Autodesk Inventor part; units mm, degrees
ref_plane "YZ Plane" through (0, 0, 0) normal (1, 0, 0) x (0, 1, 0)
ref_plane "XZ Plane" through (0, 0, 0) normal (0, 1, 0) x (-1, 0, 0)
ref_plane "XY Plane" through (0, 0, 0) normal (0, 0, 1) x (1, 0, 0)
sketch "Sketch1" plane through (0, 0, 0) normal (0, 0, 1) x (1, 0, 0)
  arc A0 (6.9595, 53) -> (8.4595, 54.5) centre (6.9595, 54.5) ccw
  line L0 (1.4595, 54.5) -> (8.4595, 54.5)
  arc A1 (1.4595, 54.5) -> (-1.5405, 51.5) centre (1.4595, 51.5) ccw
  line L1 (-1.5405, -51.5) -> (-1.5405, 51.5)
  arc A2 (-1.5405, -51.5) -> (1.4595, -54.5) centre (1.4595, -51.5) ccw
  line L2 (8.4595, -54.5) -> (1.4595, -54.5)
  arc A3 (8.4595, -54.5) -> (6.9595, -53) centre (6.9595, -54.5) ccw
  line L3 (1.4595, -53) -> (6.9595, -53)
  arc A4 (-0.0405, -51.5) -> (1.4595, -53) centre (1.4595, -51.5) ccw
  line L4 (-0.0405, 51.5) -> (-0.0405, -51.5)
  arc A5 (1.4595, 53) -> (-0.0405, 51.5) centre (1.4595, 51.5) ccw
  line L5 (6.9595, 53) -> (1.4595, 53)
  arc A6 (1.4595, 54.1) -> (-1.1405, 51.5) centre (1.4595, 51.5) ccw construction
  line L6 (1.4595, 54.1) -> (26.2595, 54.1)
  line L7 (-1.1405, 51.5) -> (-1.1405, -51.5)
  arc A7 (-1.1405, -51.5) -> (1.4595, -54.1) centre (1.4595, -51.5) ccw construction
  line L8 (1.4595, -54.1) -> (26.2595, -54.1)
  line L9 (-1.1405, -51.5) -> (1.4595, -54.1)
  line L10 (1.4595, 54.1) -> (-1.1405, 51.5)
  line L11 (26.2595, 54.1) -> (28.8595, 51.5)
  line L12 (28.8595, 51.5) -> (28.8595, -51.5)
  line L13 (28.8595, -51.5) -> (26.2595, -54.1)
  point P0 (0, 0)
  dimension "d0" = 0.4
  dimension "d1" = 30
extrude "Extrusion1" add sketch "Sketch1" along normal blind 1.8 contours L5 A5 L4 A4 L3 A3 L8 L9 L7 L10 L6 A0 | A0 L6 L11 L12 L13 L8 A3 L3 A4 L4 A5 L5
properties part number "multiplier_pcb" material "Phenolic Resin"
Here's how the part is built. I have some questions about the finished solid (model axes, mm). Round coordinates to 2 decimals unless told otherwise and drop trailing zeros.
1. If I drill on probe 1 along Y at (x, z) = (27.5, 0.35); probe 2 along Y at (x, z) = (0.75, 1.1), over which ranges is the centre line in solid material (lowest first)?
Answers:
probe 1: y = -52.86 to 52.86
probe 2: y = -53.39 to 53.39
2. Thinking about a two-plate mould opening in Z: for faces 1 (the face through (0.14, -52.78, 0.89)), 2 (the face through (14, 1, 0)), 3 (the face through (14, 1, 1.8)), which applies, released by +Z, released by -Z, zero draft, split by the parting line, or undercut?
Answers:
face 1: zero draft
face 2: released by -Z
face 3: released by +Z
3. Will this pin go through, and if not, where does the flat tip stop? pin 1 (10 mm diameter, centred on x = 7.5, y = -25.5, fed in from -Z).
Answers:
pin 1: stops at z = 0
